Verification items for this drawing (mm, ordinates from the low corner). A direction names the side the tool comes from. Give positions to 0.01 mm unless a question says otherwise; leave off trailing zeros. Loops run counter-clockwise (first coordinate to the right, second up) from the corner with the lowest first, then second, coordinate; pieces in that order, holes last. Notation, with made-up numbers: M 20.25,88 L 47.25,88 A20 cw 47.25,126 Z; hole C -14.75,-1 d1. An arc over 180 degrees is marked long. Write each question's results on one line, items separated by ' | '. Start each with the question number.
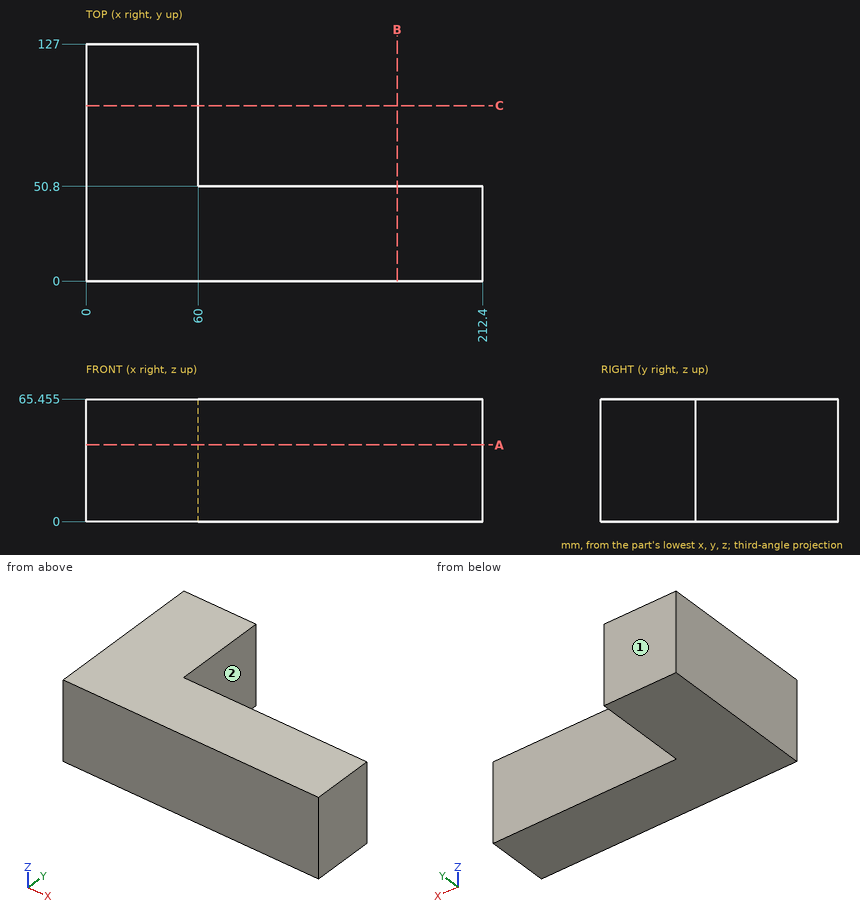
1. Set-up check for the marked faces 1 and 2: record each of +Z, -Z, +X, -X, +Y, -Y from which the full face is reachable in a straight line by a thin tool's end or side.
2. Depth check by flat-ended pin: pin 1 Ø8 at (y, z) = (98, 42) entering from +X. Enter the tip coordinate at first touch or a pass-through.
3. Section check C-C, the plane y = 94. Record the boundary of the cut face in (x, z) (1 decimal).
4. Thickness scan on probe 1 along Y at (x, z) = (127.5, 10); probe 2 along X at (y, z) = (92, 57). Record the ranges inside material, lowest first.
5. Section check B-B, the plane x = 166.5. Record the boundary of the cut face in (y, z) (1 decimal).
6. Section check A-A, the plane z = 41. Record the boundary of the cut face in (x, y).
Filled sheet:
1) face 1: +Z, -Z, +X, -X, +Y | face 2: +Z, -Z, +X, +Y
2) pin 1: x = 60
3) outline: M 0,0 L 60,0 L 60,65.5 L 0,65.5 Z
4) probe 1: 0 to 50.8 | probe 2: 0 to 60
5) outline: M 0,0 L 50.8,0 L 50.8,65.5 L 0,65.5 Z
6) outline: M 0,0 L 212.4,0 L 212.4,50.8 L 60,50.8 L 60,127 L 0,127 Z
